Geometry check sheet. Reference: the model listing, model coordinates, mm. A direction names the side the tool comes from. Round coordinates to 2 decimals unless told otherwise and drop trailing zeros. Order: outer loops, then holes, each group sorted by start corner. A loop starts at its lowest first (then second) coordinate and runs counter-clockwise, first axis right, second up. Notation, with made-up numbers: (-2, 32) -> (32, 32) arc R32 cw to (32, 67) -> close; hole circle Ø11 at (-4, 76.25). An arc over 180 degrees is marked (long way). Use a Markdown table: item, result. Add a question column.
Item 1: Sectioned sample at A-A, the plane x = 25.4. Record the cut outline in (y, z) (3 decimals).
Item 2: Sectioned sample at C-C, the plane z = 0.95. Record the cut outline in (x, y) (3 decimals), and give its area (3 significant figures).
Item 3: Sectioned sample at D-D, the plane y = -2. Record the cut outline in (x, z), and give its area (3 significant figures).
Item 4: Material ranges on probe 1 along Y at (x, z) = (25.4, 1) (3 decimals); probe 2 along Y at (x, z) = (47, 2.2) (3 decimals); probe 3 along X at (y, z) = (5.25, 1) (3 decimals), recorded low to high. Write a range as [from, to].
Item 5: Gauge pin test, flat ends, axial feed: pin 1 Ø1.5 at (y, z) = (10.5, 2) entering from +X; pin 2 Ø3 at (x, y) = (46.5, 0.5) entering from -Z. Record the tip position at first contact, or that the pin passes through.
Item 6: Set-up check for faces 1 (the flat face through (29, 0, 1)), 2 (the flat face through (45.898, 10, 1)), 3 (the flat face through (48, 0, 1)): record each of +Z, -Z, +X, -X, +Y, -Y from which the full face is reachable in a straight line by a thin tool's end or side.
Item 7: Sectioned sample at B-B, the plane y = 5. Record the cut outline in (x, z) (3 decimals).
Item 8: Mould release check, pull along X, two halves, no side actions. Record for faces 4 (the cylindrical face through (22.467, 7.794, 1.478)), 5 (the flat face through (35, 5, 0)), 6 (the flat face through (45.898, 2, 1)): pulls with the +X half, pulls with the -X half, needs draft (parallel to the pull), parting line crosses it, or undercut.
from build123d import *

# Parameters (mm, degrees)
SKETCH1_R           = 3.175
BOSS_EXTRUDE1_DEPTH = 2.9972


with BuildPart() as part:
    # Sketch1 → Boss-Extrude1 (new body)
    # profile 1 of 2: a face of its own
    with BuildSketch(Plane.XY):
        Polygon((45.8978, 0), (50.8, 0), (50.8, -2.9972), (38.1, -2.9972), (38.1, 0), align=None)
    # profile 2 of 2: a face of its own
    with BuildSketch(Plane.XY):
        with BuildLine():
            ThreePointArc((19.05, 9.525), (19.793948776, 11.321051224), (21.59, 12.065))
            Line((21.59, 12.065), (45.8978, 12.065))
            Line((45.8978, 12.065), (45.8978, 8.89))
            Line((45.8978, 8.89), (48.895, 8.89))
            Line((48.895, 8.89), (48.895, 4.445))
            Line((48.895, 4.445), (45.8978, 4.445))
            Line((45.8978, 4.445), (45.8978, 0))
            Line((45.8978, 0), (38.1, 0))
            Line((38.1, 0), (19.05, 0))
            Line((19.05, 0), (19.05, 9.525))
        make_face()
        with Locations(Location((25.4, 6.5778, 0), (0, 0, 180))):
            Circle(SKETCH1_R, mode=Mode.SUBTRACT)
    extrude(amount=BOSS_EXTRUDE1_DEPTH)


solid = part.part
Found:
| question | item | result |
|---|---|---|
| 1 | outline | (0, 0) -> (3.403, 0) -> (3.403, 2.997) -> (0, 2.997) -> close; (9.753, 0) -> (12.065, 0) -> (12.065, 2.997) -> (9.753, 2.997) -> close |
| 2 | outline | (19.05, 0) -> (38.1, 0) -> (38.1, -2.997) -> (50.8, -2.997) -> (50.8, 0) -> (45.898, 0) -> (45.898, 4.445) -> (48.895, 4.445) -> (48.895, 8.89) -> (45.898, 8.89) -> (45.898, 12.065) -> (21.59, 12.065) arc R2.54 ccw to (19.05, 9.525) -> close; hole circle Ø6.35 at (25.4, 6.578) |
| 2 | area | 342 mm2 |
| 3 | outline | (38.1, 0) -> (50.8, 0) -> (50.8, 3) -> (38.1, 3) -> close |
| 3 | area | 38.1 mm2 |
| 4 | probe 1 | y = [0, 3.403], [9.753, 12.065] |
| 4 | probe 2 | y = [-2.997, 0], [4.445, 8.89] |
| 4 | probe 3 | x = [19.05, 22.516], [28.284, 48.895] |
| 5 | pin 1 | stops at x = 45.9 |
| 5 | pin 2 | stops at z = 0 |
| 6 | face 1 | +Z, -Z, -X, -Y |
| 6 | face 2 | +Z, -Z, +X, +Y |
| 6 | face 3 | +Z, -Z, +X |
| 7 | outline | (19.05, 0) -> (22.645, 0) -> (22.645, 2.997) -> (19.05, 2.997) -> close; (28.155, 0) -> (48.895, 0) -> (48.895, 2.997) -> (28.155, 2.997) -> close |
| 8 | face 4 | undercut |
| 8 | face 5 | needs draft |
| 8 | face 6 | pulls with the +X half |
